Read the model definition and answer for the solid it produces. Units are mm, in the model's axes. Face numbers are marked on the shaded views. Coordinates: 2 decimals unless noted, no trailing zeros. Write each loop counter-clockwise with the first axis right and the second up, starting at its lowest first coordinate (ties: lowest second). Pieces come first, ordered by that corner, then holes. Notation, with made-up numbers: (61.25, 27) -> (119.25, 27) arc R20 cw to (119.25, 39) -> close; hole circle Ø11 at (71.25, 49). An arc over 180 degrees is marked (long way). Return JSON: item names as keys, results as strings.
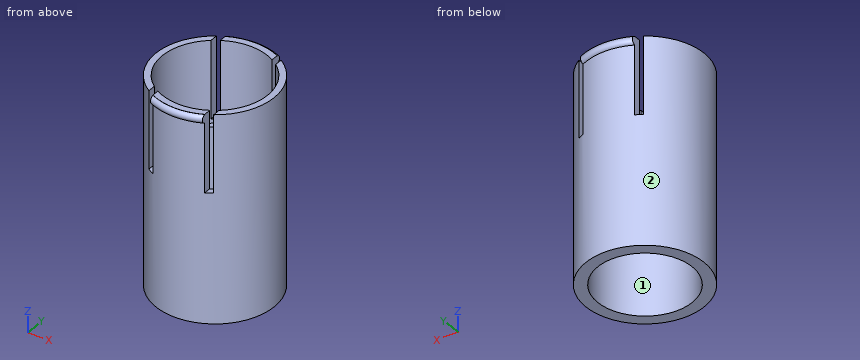
from build123d import *

# Parameters (mm, degrees)
BOX_W                    = 3
BOX_H                    = 90
BOX_DEPTH                = 40
BOX001_W                 = 3
BOX001_H                 = 90
BOX001_DEPTH             = 40
TORUS_R                  = 2
TORUS_ANGLE              = 60
TORUS_PLACEMENT_ANGLE    = 60
TORUS001_R               = 2
TORUS001_ANGLE           = 60
TORUS001_PLACEMENT_ANGLE = 240
CYLINDER001_R            = 24.5
CYLINDER001_DEPTH        = 55
CYLINDER002_R            = 24.5
CYLINDER002_DEPTH        = 60
CYLINDER008_R            = 22
CYLINDER008_DEPTH        = 90
CYLINDER_R               = 27.5
CYLINDER_DEPTH           = 96


with BuildPart() as cube:
    # Box → Box (new body)
    with BuildSketch(Plane(origin=(12, -40, 60), x_dir=(1, 0, 0), z_dir=(0, 0, 1))):
        with Locations((1.5, 45)):
            Rectangle(BOX_W, BOX_H)
    extrude(amount=BOX_DEPTH)


with BuildPart() as fusion002:
    # Box001 → Box001 (new body)
    with BuildSketch(Plane(origin=(-15, -40, 60), x_dir=(1, 0, 0), z_dir=(0, 0, 1))):
        with Locations((1.5, 45)):
            Rectangle(BOX001_W, BOX001_H)
    extrude(amount=BOX001_DEPTH)

    # Fusion002: union Cube
    add(cube.part)


with BuildPart() as torus:
    # Torus → Torus (revolve)
    with BuildSketch(Plane.XZ):
        with Locations((27, 0)):
            Circle(TORUS_R)
    revolve(axis=Axis((0, 0, 0), (0, 0, 1)), revolution_arc=TORUS_ANGLE)


with BuildPart() as torus_1:
    # Torus placement: moved
    add(torus.part.moved(Location((0, 0, 94))).rotate(Axis((0, 0, 94), (0, 0, 1)), TORUS_PLACEMENT_ANGLE))


with BuildPart() as torus001:
    # Torus001 → Torus001 (revolve)
    with BuildSketch(Plane.XZ):
        with Locations((27, 0)):
            Circle(TORUS001_R)
    revolve(axis=Axis((0, 0, 0), (0, 0, 1)), revolution_arc=TORUS001_ANGLE)


with BuildPart() as torus001_1:
    # Torus001 placement: moved
    add(torus001.part.moved(Location((0, 0, 94))).rotate(Axis((0, 0, 94), (0, 0, 1)), TORUS001_PLACEMENT_ANGLE))


with BuildPart() as cylinder001:
    # Cylinder001 → Cylinder001 (new body)
    with BuildSketch(Plane.XY.offset(58)):
        Circle(CYLINDER001_R)
    extrude(amount=CYLINDER001_DEPTH)


with BuildPart() as fusion:
    # Cylinder002 → Cylinder002 (new body)
    with BuildSketch(Plane.XY.offset(58)):
        Circle(CYLINDER002_R)
    extrude(amount=CYLINDER002_DEPTH)

    # Fusion: union Cylinder001
    add(cylinder001.part)


with BuildPart() as cylinder008:
    # Cylinder008 → Cylinder008 (new body)
    with BuildSketch(Plane.XY):
        Circle(CYLINDER008_R)
    extrude(amount=CYLINDER008_DEPTH)


with BuildPart() as main_bit:
    # Cylinder → Cylinder (new body)
    with BuildSketch(Plane.XY):
        Circle(CYLINDER_R)
    extrude(amount=CYLINDER_DEPTH)

    # Cut: cut Cylinder008
    add(cylinder008.part, mode=Mode.SUBTRACT)

    # Cut004: cut Fusion
    add(fusion.part, mode=Mode.SUBTRACT)

    # Fusion001: union Torus, Torus001
    add(torus_1.part)
    add(torus001_1.part)

    # Cut007: cut Fusion002
    add(fusion002.part, mode=Mode.SUBTRACT)


solid = main_bit.part
1. The part is cut by section B-B (x = 0). Determine the outline of the cut face in (y, z).
Taken from the geometry:
{"outline": "(-27.5, 0) -> (-22, 0) -> (-22, 58) -> (-24.5, 58) -> (-24.5, 96) -> (-27.5, 96) -> (-27.5, 95.94) arc R2 ccw to (-27.5, 92.06) -> close; (22, 0) -> (27.5, 0) -> (27.5, 92.06) arc R2 ccw to (27.5, 95.94) -> (27.5, 96) -> (24.5, 96) -> (24.5, 58) -> (22, 58) -> close"}
2. The part is cut by section A-A (y = 0). Determine the outline of the cut face in (x, z), then the cut area to 3 significant figures.
Taken from the geometry:
{"outline": "(-27.5, 0) -> (-22, 0) -> (-22, 58) -> (-24.5, 58) -> (-24.5, 96) -> (-27.5, 96) -> close; (22, 0) -> (27.5, 0) -> (27.5, 96) -> (24.5, 96) -> (24.5, 58) -> (22, 58) -> close", "area": "866 mm2"}
3. Flat-ended cylindrical pins translate along their axes: pin 1 Ø2.5 at (x, y) = (13.5, -21.5) entering from +Z; pin 2 Ø3.5 at (x, y) = (-13, 22.5) entering from +Z; pin 3 Ø2 at (x, z) = (9, 82.5) entering from +Y; pin 4 Ø1.8 at (y, z) = (21.5, 77.5) entering from +X. Find the tip coordinate at first contact, or state that the pin passes through.
Taken from the geometry:
{"pin 1": "stops at z = 60", "pin 2": "stops at z = 96", "pin 3": "stops at y = 26.31", "pin 4": "stops at x = 18.22"}
4. The part is cut by section C-C (z = 70). Determine the outline of the cut face in (x, y).
Taken from the geometry:
{"outline": "(-15, -23.05) -> (-15, -19.37) arc R24.5 cw to (-15, 19.37) -> (-15, 23.05) arc R27.5 ccw to start; (-12, -24.74) arc R27.5 ccw to (12, -24.74) -> (12, -21.36) arc R24.5 cw to (-12, -21.36) -> close; (-12, 21.36) arc R24.5 cw to (12, 21.36) -> (12, 24.74) arc R27.5 ccw to (-12, 24.74) -> close; (15, -23.05) arc R27.5 ccw to (15, 23.05) -> (15, 19.37) arc R24.5 cw to (15, -19.37) -> close"}
5. For a pull along Y with two mould halves and no side action, classify the marked faces 1 and 2 as +Y half, -Y half, draft (parallel to the pull), parting line (faces both ways), or undercut.
Taken from the geometry:
{"face 1": "undercut", "face 2": "parting line"}
6. The part is cut by section D-D (z = 18.5). Determine the outline of the cut face in (x, y).
Taken from the geometry:
{"outline": "circle Ø55 at (0, 0); hole circle Ø44 at (0, 0)"}
7. Consider L1, parallel to X at y = 0, z = 23.5; L2, parallel to Y at x = 0, z = 66. Determine where each line is inside the solid, lowest interval first.
Taken from the geometry:
{"L1": "x = -27.5 to -22, 22 to 27.5", "L2": "y = -27.5 to -24.5, 24.5 to 27.5"}
